Check sheet for the modelled part. Datum: model origin and axes. Units: mm. A direction names the side the tool comes from. Coordinates: 2 decimals unless noted, no trailing zeros. Loops run counter-clockwise (first coordinate to the right, second up) from the corner with the lowest first, then second, coordinate; pieces in that order, holes last. Notation, with made-up numbers: M 52.25,0.5 L 96.25,0.5 A26 cw 96.25,31.5 Z; hole C 66,-17 d9. An arc over 180 degrees is marked long. Write each question's results on one line, items separated by ' | '. Start each with the question number.
from build123d import *

# Parameters (mm, degrees)
BOSS_EXTRUDE1_DEPTH = 4
CUT_EXTRUDE1_DEPTH  = 10


with BuildPart() as part:
    # Sketch1 → Boss-Extrude1 (new body)
    with BuildSketch(Plane(origin=(0, 0, 0), x_dir=(1, 0, 0), z_dir=(0, 1, 0))):
        Polygon((-10.4, 13.35), (-10.4, 11.35), (-14.4, 11.35), (-14.4, 7.35), (-10.4, 7.35), (-10.4, 3.35), (-14.4, 3.35), (-14.4, -0.65), (-10.4, -0.65), (-10.4, -4.65), (-14.4, -4.65), (-14.4, -8.65), (-10.4, -8.65), (-10.4, -12.65), (-14.4, -12.65), (-14.4, -16.65), (-10.4, -16.65), (-10.4, -20.65), (-14.4, -20.65), (-14.4, -24.65), (-10.4, -24.65), (-10.4, -28.65), (-14.4, -28.65), (-14.4, -32.65), (-10.4, -32.65), (-10.4, -36.65), (-14.4, -36.65), (-14.4, -40.65), (-10.4, -40.65), (-10.4, -44.65), (79.6, -44.65), (79.6, -40.65), (83.6, -40.65), (83.6, -36.65), (79.6, -36.65), (79.6, -24.65), (83.6, -24.65), (83.6, -20.65), (79.6, -20.65), (79.6, -8.65), (83.6, -8.65), (83.6, -4.65), (79.6, -4.65), (79.6, 7.35), (83.6, 7.35), (83.6, 11.35), (79.6, 11.35), (79.6, 13.35), align=None)
    extrude(amount=-BOSS_EXTRUDE1_DEPTH)

    # Sketch2 → Cut-Extrude1 (cut)
    with BuildSketch(Plane(origin=(0, 0, 0), x_dir=(1, 0, 0), z_dir=(0, 1, 0))):
        with BuildLine():
            Line((3.269007855, 9.35), (29.6, 9.35))
            ThreePointArc((29.6, 9.35), (31.014213562, 8.764213562), (31.6, 7.35))
            Line((31.6, 7.35), (31.6, -7.255623888))
            ThreePointArc((31.6, -7.255623888), (30.61482352, -8.979031334), (28.629866776, -9.004578298))
            Line((28.629866776, -9.004578298), (2.29887463, 5.60104559))
            ThreePointArc((2.29887463, 5.60104559), (1.332786171, 7.851044499), (3.269007855, 9.35))
        make_face()
        with BuildLine():
            ThreePointArc((-6.4, 2.455623888), (-5.41482352, 4.179031334), (-3.429866776, 4.204578298))
            Line((-3.429866776, 4.204578298), (22.90112537, -10.40104559))
            ThreePointArc((22.90112537, -10.40104559), (23.867213829, -12.651044499), (21.930992145, -14.15))
            Line((21.930992145, -14.15), (-4.4, -14.15))
            ThreePointArc((-4.4, -14.15), (-5.814213562, -13.564213562), (-6.4, -12.15))
            Line((-6.4, -12.15), (-6.4, 2.455623888))
        make_face()
        with BuildLine():
            ThreePointArc((-6.4, -19.15), (-5.814213562, -17.735786438), (-4.4, -17.15))
            Line((-4.4, -17.15), (21.930992145, -17.15))
            ThreePointArc((21.930992145, -17.15), (23.867213829, -18.648955501), (22.90112537, -20.89895441))
            Line((22.90112537, -20.89895441), (-3.429866776, -35.504578298))
            ThreePointArc((-3.429866776, -35.504578298), (-5.41482352, -35.479031334), (-6.4, -33.755623888))
            Line((-6.4, -33.755623888), (-6.4, -19.15))
        make_face()
        with BuildLine():
            Line((31.6, -38.65), (31.6, -24.044376112))
            ThreePointArc((31.6, -24.044376112), (30.61482352, -22.320968666), (28.629866776, -22.295421702))
            Line((28.629866776, -22.295421702), (2.29887463, -36.90104559))
            ThreePointArc((2.29887463, -36.90104559), (1.332786171, -39.151044499), (3.269007855, -40.65))
            Line((3.269007855, -40.65), (29.6, -40.65))
            ThreePointArc((29.6, -40.65), (31.014213562, -40.064213562), (31.6, -38.65))
        make_face()
        with BuildLine():
            Line((65.930992145, -40.65), (39.6, -40.65))
            ThreePointArc((39.6, -40.65), (38.185786438, -40.064213562), (37.6, -38.65))
            Line((37.6, -38.65), (37.6, -24.044376112))
            ThreePointArc((37.6, -24.044376112), (38.58517648, -22.320968666), (40.570133224, -22.295421702))
            Line((40.570133224, -22.295421702), (66.90112537, -36.90104559))
            ThreePointArc((66.90112537, -36.90104559), (67.867213829, -39.151044499), (65.930992145, -40.65))
        make_face()
        with BuildLine():
            ThreePointArc((75.6, -33.755623888), (74.61482352, -35.479031334), (72.629866776, -35.504578298))
            Line((72.629866776, -35.504578298), (46.29887463, -20.89895441))
            ThreePointArc((46.29887463, -20.89895441), (45.332786171, -18.648955501), (47.269007855, -17.15))
            Line((47.269007855, -17.15), (73.6, -17.15))
            ThreePointArc((73.6, -17.15), (75.014213562, -17.735786438), (75.6, -19.15))
            Line((75.6, -19.15), (75.6, -33.755623888))
        make_face()
        with BuildLine():
            ThreePointArc((75.6, -12.15), (75.014213562, -13.564213562), (73.6, -14.15))
            Line((73.6, -14.15), (47.269007855, -14.15))
            ThreePointArc((47.269007855, -14.15), (45.332786171, -12.651044499), (46.29887463, -10.40104559))
            Line((46.29887463, -10.40104559), (72.629866776, 4.204578298))
            ThreePointArc((72.629866776, 4.204578298), (74.61482352, 4.179031334), (75.6, 2.455623888))
            Line((75.6, 2.455623888), (75.6, -12.15))
        make_face()
        with BuildLine():
            Line((37.6, 7.35), (37.6, -7.255623888))
            ThreePointArc((37.6, -7.255623888), (38.58517648, -8.979031334), (40.570133224, -9.004578298))
            Line((40.570133224, -9.004578298), (66.90112537, 5.60104559))
            ThreePointArc((66.90112537, 5.60104559), (67.867213829, 7.851044499), (65.930992145, 9.35))
            Line((65.930992145, 9.35), (39.6, 9.35))
            ThreePointArc((39.6, 9.35), (38.185786438, 8.764213562), (37.6, 7.35))
        make_face()
    extrude(amount=-CUT_EXTRUDE1_DEPTH, mode=Mode.SUBTRACT)


solid = part.part
Item 1: Section check D-D (y = -2.5). State how many separate pieces and enclosed holes the cut face has, plus the area to 3 significant figures.
Item 2: Release check for a two-part mould opening along Z. For faces 1 (the face through (23.876, -1.972, 12.615)), 2 (the face through (-14.4, -2, 39)), 3 (the face through (35, -2, -13.35)) record: +Z half, -Z half, draft (parallel to the pull), parting line (faces both ways), or undercut.
Item 3: Section check C-C (x = 49.5). Record the cut outline in (y, z).
Item 4: Thickness scan on line 1 (Z direction, x = 51, y = -1.9); line 2 (X direction, y = -3.8, z = 1); line 3 (Z direction, x = 20.5, y = -2.95) (3 decimals). Record the ranges inside material, lowest first.
Item 5: Tool access check on faces 4 (the face through (82, -2, -7.35)), 5 (the face through (37.6, -2, 0)), 6 (the face through (-12, -2, 28.65)). Record the directions out of +Z, -Z, +X, -X, +Y, -Y that give a thin tool (end or side, any length) a straight path to the whole face; none if there is none.
Item 6: Section check B-B (z = 2.5). Record the cut outline in (x, y), plus the area to 3 significant figures.
Item 7: Depth check by flat-ended pin: P1, Ø1.2, axis at y = -2.5, z = 43, coming from the +X side; P2, Ø1.2, axis at x = -13, y = -2, coming from the -Z side; P3, Ø2, axis at x = 82.5, y = -2, coming from the +Z side. Enter the tip coordinate at first touch or a pass-through.
Item 8: Section check A-A (x = 25). Record the cut outline in (y, z), plus the area to 3 significant figures.
Computed values:
1) separate pieces: 1 | enclosed holes: 8 | area: 2,620 mm²
2) face 1: undercut | face 2: draft | face 3: -Z half
3) outline: M -4,-13.35 L 0,-13.35 L 0,-9.35 L -4,-9.35 Z; M -4,4.05 L 0,4.05 L 0,8.63 L -4,8.63 Z; M -4,14.15 L 0,14.15 L 0,17.15 L -4,17.15 Z; M -4,22.67 L 0,22.67 L 0,27.25 L -4,27.25 Z; M -4,40.65 L 0,40.65 L 0,44.65 L -4,44.65 Z
4) line 1: z = -13.35 to -9.35, 3.22 to 7.79, 14.15 to 17.15, 23.51 to 28.08, 40.65 to 44.65 | line 2: x = -10.4 to -6.4, 5.95 to 14.2, 31.6 to 37.6, 55 to 63.25, 75.6 to 79.6 | line 3: z = -13.35 to -9.35, 4.495 to 9.069, 14.15 to 17.15, 22.231 to 26.805, 40.65 to 44.65
5) face 4: +X, +Y, -Y | face 5: +Y, -Y | face 6: -X, +Y, -Y
6) outline: M -10.4,-4 L -6.4,-4 L -6.4,0 L -10.4,0 Z; M 8.66,-4 L 16.9,-4 L 16.9,0 L 8.66,0 Z; M 31.6,-4 L 37.6,-4 L 37.6,0 L 31.6,0 Z; M 52.3,-4 L 60.54,-4 L 60.54,0 L 52.3,0 Z; M 75.6,-4 L 79.6,-4 L 79.6,0 L 75.6,0 Z | area: 122 mm²
7) P1: stops at x = 79.6 | P2: stops at z = -11.35 | P3: stops at z = 40.65
8) outline: M -4,-13.35 L 0,-13.35 L 0,-9.35 L -4,-9.35 Z; M -4,6.99 L 0,6.99 L 0,24.31 L -4,24.31 Z; M -4,40.65 L 0,40.65 L 0,44.65 L -4,44.65 Z | area: 101 mm²
